Could you check a few things on this model? Use its own coordinates, in mm. A direction names the side the tool comes from. Round coordinates to 2 decimals unless told otherwise and drop trailing zeros. Write each loop counter-clockwise with the first axis right and the second up, starting at its lowest first coordinate (ties: lowest second). Pieces come first, ordered by that corner, then holes. Notation, with made-up numbers: (-1.5, 30.25) - (22.5, 30.25) arc R14 cw to (22.5, 50.25) - close; hole circle Ø5 at (16, 88.25). An arc over 180 degrees is marked (long way). Write each question's results on one line, items separated by ' | '. Start each with the question number.
(1) Imagine slicing it at B-B on x = 78. Write out the boundary of the cut face in (y, z), then the cut area to 4 significant figures.
(2) Imagine slicing it at A-A on x = 11.5. Write out the boundary of the cut face in (y, z), then the cut area to 3 significant figures.
(3) Thinking about a two-plate mould opening in Y: for faces 5 (the flat face through (18, 12, 8.5)), 6 (the flat face through (18, 2, 12)), 7 (the flat face through (43, 35.25, 6)), 8 (the flat face through (42, -35.25, 6)), which applies, +Y half, -Y half, draft (parallel to the pull), parting line (faces both ways), or undercut?
(4) Imagine slicing it at D-D on y = 0. Write out the boundary of the cut face in (x, z), then the cut area to 3 significant figures.
(5) On a 3-axis mill with a long thin cutter (end or side, diameter ignored), from which of +Z, -Z, +X, -X, +Y, -Y can I reach the whole of each face in a straight line? I mean faces 1 (the flat face through (15.7, 9.6, 9.9)), 2 (the flat face through (4, 3.5, 6)), 3 (the flat face through (36.59, -14.84, 5.92)), 4 (the flat face through (0, -20, 6)). Say none if no direction works.
(6) Please list where these lines run through material, in increasing order: line 1 (Y direction, x = 11.5, z = 2.5); line 2 (Y direction, x = 68, z = 7.5); line 3 (Y direction, x = 24.5, z = 9.25). Write a range as [from, to].
(7) For P1, Ø1.5, axis at x = 31, y = -0.5, coming from the -Z side (1 decimal); P2, Ø5, axis at x = 19.5, y = -11.5, coming from the +Z side; P3, Ø3.5, axis at x = 25.5, y = 12.5, coming from the +Z side, each with a flat end and sliding along its axis, tell me the tip position at first contact or that it passes through.
(8) Imagine slicing it at C-C on z = 2.75. Write out the boundary of the cut face in (x, y), then the cut area to 3 significant figures.
```python
from build123d import *

# Parameters (mm, degrees)
F1_DEPTH = 12
F2_W     = 8
F2_H     = 7
F3_DEPTH = 12
F4_R     = 6.5
F5_DEPTH = 12
F6_SIZE  = 1.5
F8_DEPTH = 40
F9_R     = 1


with BuildPart() as f1:
    # F0 (on Top) → F1 (new body)
    with BuildSketch(Plane.XY):
        Polygon((85, 35.25), (0, 35.25), (0, -35.25), (85, -35.25), (85, -21.25), (43, -21.25), (30, -8.25), (30, 8.25), (43, 21.25), (85, 21.25), align=None)
    extrude(amount=F1_DEPTH)

    # F2 (on Top) → F3 (cut)
    with BuildSketch(Plane.XY):
        with Locations((4, 0)):
            Rectangle(F2_W, F2_H)
    extrude(amount=F3_DEPTH, mode=Mode.SUBTRACT)

    # F4 (on Top) → F5 (cut)
    with BuildSketch(Plane.XY):
        with Locations((11.5, 0)):
            Circle(F4_R)
    extrude(amount=F5_DEPTH, mode=Mode.SUBTRACT)

    # F6
    f6_edges = [f1.edges().sort_by_distance(p)[0] for p in [
        (42.5, -35.25, 12),
        (42.5, 35.25, 12),
        (42.5, -35.25, 0),
        (42.5, 35.25, 0),
        (0, 3.5, 6),
        (0, -3.5, 6),
    ]]
    chamfer(f6_edges, length=F6_SIZE)

    # F7 (on Right) → F8 (cut)
    with BuildSketch(Plane.YZ):
        Polygon((-10, 8.5), (-9, 12), (-15.5, 12), (-14.5, 8.5), align=None)
        Polygon((14.5, 8.5), (15.5, 12), (9, 12), (10, 8.5), align=None)
    extrude(amount=F8_DEPTH, mode=Mode.SUBTRACT)

    # F9
    f9_edges = [f1.edges().sort_by_distance(p)[0] for p in [
        (18.625, 15.5, 12),
        (18.625, -15.5, 12),
        (15.375, -9, 12),
        (15.375, 9, 12),
    ]]
    fillet(f9_edges, radius=F9_R)


solid = f1.part
```
Response:
1) outline: (-35.25, 1.5) - (-33.75, 0) - (-21.25, 0) - (-21.25, 12) - (-33.75, 12) - (-35.25, 10.5) - close; (21.25, 0) - (33.75, 0) - (35.25, 1.5) - (35.25, 10.5) - (33.75, 12) - (21.25, 12) - close | area: 331.5 mm²
2) outline: (-35.25, 1.5) - (-33.75, 0) - (-6.5, 0) - (-6.5, 12) - (-8.25, 12) arc R1 ccw to (-9.21, 11.27) - (-10, 8.5) - (-14.5, 8.5) - (-15.29, 11.27) arc R1 ccw to (-16.25, 12) - (-33.75, 12) - (-35.25, 10.5) - close; (6.5, 0) - (33.75, 0) - (35.25, 1.5) - (35.25, 10.5) - (33.75, 12) - (16.25, 12) arc R1 ccw to (15.29, 11.27) - (14.5, 8.5) - (10, 8.5) - (9.21, 11.27) arc R1 ccw to (8.25, 12) - (6.5, 12) - close | area: 647 mm²
3) face 5: undercut | face 6: draft | face 7: +Y half | face 8: -Y half
4) outline: (18, 0) - (30, 0) - (30, 12) - (18, 12) - close | area: 144 mm²
5) face 1: +Z, +X, -X | face 2: +Z, -Z, -X | face 3: +Z, -Z, +X | face 4: +Z, -Z, -X, +Y, -Y
6) line 1: [-35.25, -6.5], [6.5, 35.25] | line 2: [-35.25, -21.25], [21.25, 35.25] | line 3: [-35.25, -14.71], [-9.79, 9.79], [14.71, 35.25]
7) P1: through | P2: z = 11.66 | P3: z = 8.5
8) outline: (0, -35.25) - (85, -35.25) - (85, -21.25) - (43, -21.25) - (30, -8.25) - (30, 8.25) - (43, 21.25) - (85, 21.25) - (85, 35.25) - (0, 35.25) - (0, 5) - (1.5, 3.5) - (6.02, 3.5) arc R6.5 cw (long way) to (6.02, -3.5) - (1.5, -3.5) - (0, -5) - close | area: 3,650 mm²
